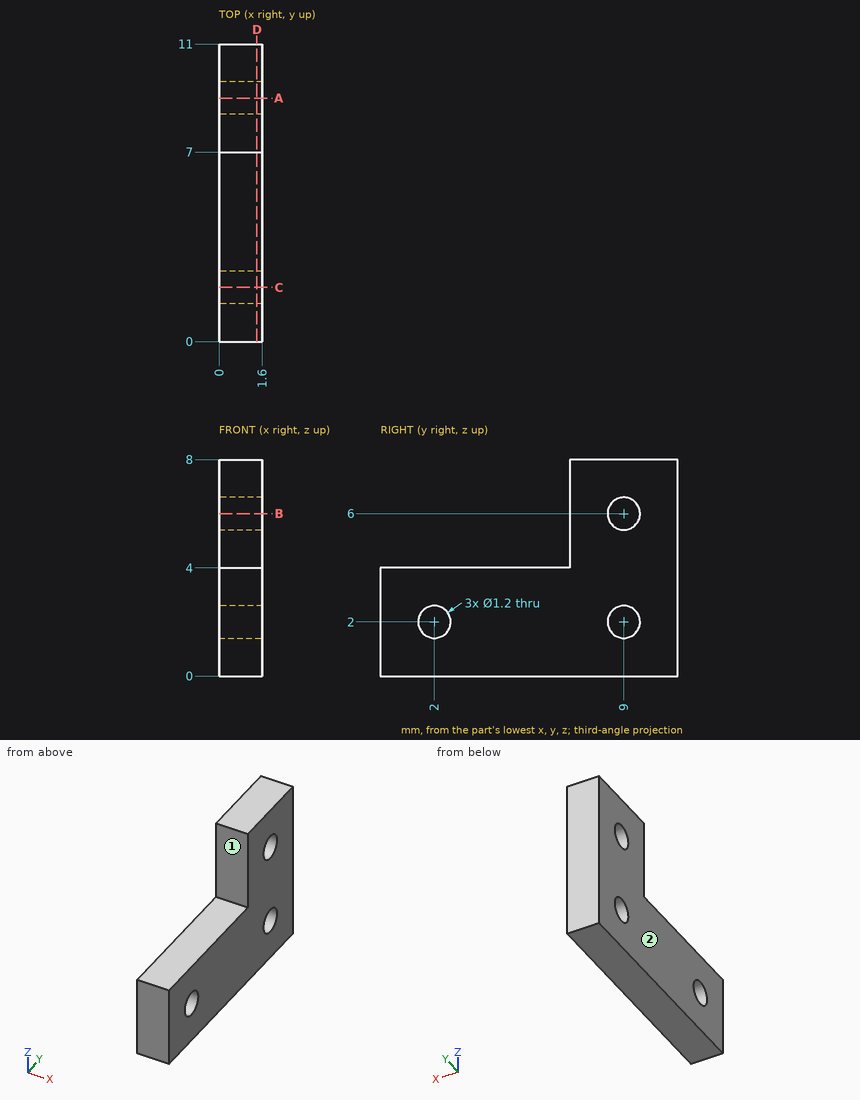
Geometry check sheet. Reference: drawing and pictorial views, mm from the part's lowest x, y, z. A direction names the side the tool comes from. Round coordinates to 2 decimals unless told otherwise and drop trailing zeros. Order: outer loops, then holes, each group sorted by start corner. A loop starts at its lowest first (then second) coordinate and runs counter-clockwise, first axis right, second up. Notation, with made-up numbers: M 4,32 L 34,32 A16 ccw 34,37 Z; hole C 23,-30 d10. An arc over 180 degrees is marked long. One line per item, written item: value. Start each with the question number.
1. Section check C-C on y = 2. Enter the section's corners in (x, z).
2. Scan lines: line 1 along Y through (x, z) = (1.2, 2); line 2 along Z through (x, y) = (0.1, 3); line 3 along Y through (x, z) = (0.6, 4.25). Record each from-to range of solid material in increasing order.
3. Section check B-B on z = 6. Enter the section's corners in (x, y).
4. Section check A-A on y = 9. Enter the section's corners in (x, z).
5. Section check D-D on x = 1.4. Enter the section's corners in (y, z), and give its area (3 significant figures).
6. Access from +Z, -Z, +X, -X, +Y, -Y to the whole of each face (thin tool, end or side, straight path). Record for the marked faces 1 and 2.
7. Gauge pin test, flat ends, axial feed: P1, Ø0.8, axis at x = 1, z = 5, coming from the -Y side; P2, Ø1.1, axis at y = 2, z = 2, coming from the +X side. Record the tip position at first contact, or that the pin passes through.
Results found:
1. outline: M 0,0 L 1.6,0 L 1.6,1.4 L 0,1.4 Z; M 0,2.6 L 1.6,2.6 L 1.6,4 L 0,4 Z
2. line 1: 0 to 1.4, 2.6 to 8.4, 9.6 to 11
2. line 2: 0 to 4
2. line 3: 7 to 11
3. outline: M 0,7 L 1.6,7 L 1.6,8.4 L 0,8.4 Z; M 0,9.6 L 1.6,9.6 L 1.6,11 L 0,11 Z
4. outline: M 0,0 L 1.6,0 L 1.6,1.4 L 0,1.4 Z; M 0,2.6 L 1.6,2.6 L 1.6,5.4 L 0,5.4 Z; M 0,6.6 L 1.6,6.6 L 1.6,8 L 0,8 Z
5. outline: M 0,0 L 11,0 L 11,8 L 7,8 L 7,4 L 0,4 Z; hole C 2,2 d1.2; hole C 9,2 d1.2; hole C 9,6 d1.2
5. area: 56.6 mm^2
6. face 1: +Z, +X, -X, -Y
6. face 2: +Z, -Z, -X, +Y, -Y
7. P1: y = 7
7. P2: through
